Input: part model. Units: mm. Frame: model coordinates. A direction names the side the tool comes from. Give positions to 0.01 mm unless a question says otherwise; leave off trailing zeros. Loops run counter-clockwise (first coordinate to the right, second up) from the corner with the lowest first, then second, coordinate; pieces in that order, holes last. Notation, with made-up numbers: (3.25, 88) - (10.25, 88) arc R12 ccw to (10.25, 94) - close; hole circle Ø6 at (61.25, -38.75). An arc over 180 degrees is marked (long way). One line per item, written item: value.
from build123d import *

# Parameters (mm, degrees)
SKETCH_1_R          = 6.5
EXTRUDE_1_DEPTH     = 20
CUT_EXTRUDE_1_DEPTH = 17
SKETCH_3_R          = 2.5
EXTRUDE_2_DEPTH     = 13
CUT_EXTRUDE_START   = -12
CUT_EXTRUDE_2_DEPTH = 12
CHAMFER_1_SIZE      = 1
CUT_EXTRUDE_3_DEPTH = 17
CHAMFER_2_SIZE      = 0.5
CHAMFER_3_SIZE      = 0.5
SKETCH_6_R          = 1.25
CUT_EXTRUDE_4_DEPTH = 10


with BuildPart() as part:
    # 草图1 → 凸台-拉伸1 (new body)
    with BuildSketch(Plane.XY):
        Circle(SKETCH_1_R)
    extrude(amount=EXTRUDE_1_DEPTH)

    # 草图2 → 切除-拉伸1 (cut)
    with BuildSketch(Plane(origin=(0, 0, 0), x_dir=(-1, 0, 0), z_dir=(0, 0, -1))):
        with BuildLine():
            Line((3.122498999, 2.5), (-3.122498999, 2.5))
            ThreePointArc((-3.122498999, 2.5), (-3.605551275, -1.732050808), (0, -4))
            ThreePointArc((0, -4), (2.828427125, -2.828427125), (4, 0))
            ThreePointArc((4, 0), (3.774254628, 1.324764885), (3.122498999, 2.5))
        make_face()
    extrude(amount=-CUT_EXTRUDE_1_DEPTH, mode=Mode.SUBTRACT)

    # 草图3 → 凸台-拉伸2 (add)
    with BuildSketch(Plane.XY.offset(20)):
        with Locations(Location((0, 0, 0), (0, 0, 180))):
            Circle(SKETCH_3_R)
    extrude(amount=EXTRUDE_2_DEPTH)

    # 草图4 → 切除-拉伸2 (cut)
    with BuildSketch(Plane.XY.offset(33).offset(CUT_EXTRUDE_START)):
        with BuildLine():
            Line((-1.5, 2), (1.5, 2))
            ThreePointArc((1.5, 2), (0, 2.5), (-1.5, 2))
        make_face()
    extrude(amount=CUT_EXTRUDE_2_DEPTH, mode=Mode.SUBTRACT)

    # 倒角1
    chamfer_1_edges = [part.edges().sort_by_distance(p)[0] for p in [
        (2.5, 0, 20),
    ]]
    chamfer(chamfer_1_edges, length=CHAMFER_1_SIZE - 0.0001)  # a hair under: the kernel refuses the full size

    # 草图5 → 切除-拉伸3 (cut)
    with BuildSketch(Plane(origin=(0, 0, 0), x_dir=(-1, 0, 0), z_dir=(0, 0, -1))):
        with BuildLine():
            Line((3.170173497, 2.6), (-3.170173497, 2.6))
            ThreePointArc((-3.170173497, 2.6), (0, -4.1), (3.170173497, 2.6))
        make_face()
    extrude(amount=-CUT_EXTRUDE_3_DEPTH, mode=Mode.SUBTRACT)

    # 倒角2
    chamfer_2_edges = [part.edges().sort_by_distance(p)[0] for p in [
        (1.118033989, -2.236067977, 33),
        (0, 2, 33),
    ]]
    chamfer(chamfer_2_edges, length=CHAMFER_2_SIZE - 0.0001)  # a hair under: the kernel refuses the full size

    # 倒角3
    chamfer_3_edges = [part.edges().sort_by_distance(p)[0] for p in [
        (-6.5, 0, 0),
        (0, -4.1, 0),
        (0, 2.6, 0),
        (-6.5, 0, 20),
    ]]
    chamfer(chamfer_3_edges, length=CHAMFER_3_SIZE)

    # 草图6 → 切除-拉伸4 (cut)
    with BuildSketch(Plane(origin=(0, 0, 0), x_dir=(1, 0, 0), z_dir=(0, 1, 0))):
        with Locations(Location((0, -6, 0), (0, 0, 90))):
            Circle(SKETCH_6_R)
    extrude(amount=CUT_EXTRUDE_4_DEPTH, mode=Mode.SUBTRACT)


solid = part.part
Item 1: Pin query (flat end, axial travel): P1, Ø3, axis at x = 1, y = 0.5, coming from the -Z side; P2, Ø1.5, axis at x = 0.5, z = 28, coming from the +Y side; P3, Ø1, axis at x = 2.5, y = 4, coming from the -Z side; P4, Ø6, axis at y = 4.5, z = 14.5, coming from the +X side. Return the tip coordinate at first contact, or that it passes through.
Verdict:
P1: stops at z = 17
P2: stops at y = 2
P3: stops at z = 0
P4: stops at x = 6.32
Item 2: Section D-D, the plane z = 30. Output: boundary loops of the cut face in (x, y), and give its area (3 significant figures).
Verdict:
outline: (-1.5, 2) arc R2.5 ccw (long way) to (1.5, 2) - close
area: 18.6 mm^2
Item 3: Draft query along Y for faces 1 (the face through (-0.075, -2.134, 32.865)), 2 (the face through (0, 4, 0)), 3 (the face through (0, -1, 17)). Return one class per face: pulls with the +Y half, pulls with the -Y half, needs draft (parallel to the pull), parting line crosses it, or undercut.
Verdict:
face 1: parting line crosses it
face 2: needs draft
face 3: undercut
Item 4: Material intervals for L1, parallel to Y at x = 0, z = 5.5; L2, parallel to Y at x = 0, z = 4.25; L3, parallel to Z at x = 4.5, y = 1.5, sorted ascending.
Verdict:
L1: y = -6.5 to -4.1
L2: y = -6.5 to -4.1, 2.6 to 6.5
L3: z = 0 to 20
Item 5: Section C-C, the plane z = 6. Output: boundary loops of the cut face in (x, y).
Verdict:
outline: (-3.17, 2.6) - (-1.25, 2.6) - (-1.25, 6.38) arc R6.5 ccw (long way) to (1.25, 6.38) - (1.25, 2.6) - (3.17, 2.6) arc R4.1 cw (long way) to start
Item 6: Access query for faces 4 (the face through (-0.05, 4.52, 7.25)), 5 (the face through (0, 2, 27)), 6 (the face through (0.1, -4.1, 8.6)). Directions: +Z, -Z, +X, -X, +Y, -Y. A direction counts if a zero-diameter tool reaches every point of the face in a straight line with its end or side. Return the directions, or none.
Verdict:
face 4: +Y
face 5: +Z, +X, -X, +Y
face 6: -Z
Item 7: Section B-B, the plane y = 0. Output: boundary loops of the cut face in (x, z), and give its area (3 significant figures).
Verdict:
outline: (-6.5, 0.5) - (-6, 0) - (-4.6, 0) - (-4.1, 0.5) - (-4.1, 17) - (4.1, 17) - (4.1, 0.5) - (4.6, 0) - (6, 0) - (6.5, 0.5) - (6.5, 19.5) - (6, 20) - (3.5, 20) - (2.5, 21) - (2.5, 32.5) - (2, 33) - (-2, 33) - (-2.5, 32.5) - (-2.5, 21) - (-3.5, 20) - (-6, 20) - (-6.5, 19.5) - close
area: 186 mm^2
